```python
from build123d import *

# Parameters (mm, degrees)
ESBO_O1_R                = 4.1
ESBO_O1_R_2              = 1.2
RESSALTO_EXTRUS_O1_DEPTH = 1
ESBO_O2_W                = 5
ESBO_O2_H                = 1
RESSALTO_EXTRUS_O2_DEPTH = 22.2
ESBO_O3_R                = 1.2
RESSALTO_EXTRUS_O3_DEPTH = 1
FILETE1_R                = 1
BODY_MOVE_COPY2_ANGLE    = 90


with BuildPart() as part:
    # Esboço1 → Ressalto-extrusão1 (new body)
    with BuildSketch(Plane(origin=(0, 0, 0), x_dir=(1, 0, 0), z_dir=(0, 1, 0))):
        with BuildLine():
            Line((-2.5, 15), (-2.5, 12.247448714))
            ThreePointArc((-2.5, 12.247448714), (-10.825317547, 6.25), (-11.856601718, -3.958660847))
            Line((-11.856601718, -3.958660847), (-14.240381057, -5.334936491))
            Line((-14.240381057, -5.334936491), (-11.740381057, -9.665063509))
            Line((-11.740381057, -9.665063509), (-9.356601718, -8.288787866))
            ThreePointArc((-9.356601718, -8.288787866), (0, -12.5), (9.356601718, -8.288787866))
            Line((9.356601718, -8.288787866), (11.740381057, -9.665063509))
            Line((11.740381057, -9.665063509), (14.240381057, -5.334936491))
            Line((14.240381057, -5.334936491), (11.856601718, -3.958660847))
            ThreePointArc((11.856601718, -3.958660847), (10.825317547, 6.25), (2.5, 12.247448714))
            Line((2.5, 12.247448714), (2.5, 15))
            Line((2.5, 15), (-2.5, 15))
        make_face()
        with Locations(Location((0, 0, 0), (0, 0, 270))):
            Circle(ESBO_O1_R, mode=Mode.SUBTRACT)
        with Locations(Location((0, 6.75, 0), (0, 0, 270))):
            Circle(ESBO_O1_R_2, mode=Mode.SUBTRACT)
        with Locations(Location((5.845671476, -3.375, 0), (0, 0, 270))):
            Circle(ESBO_O1_R_2, mode=Mode.SUBTRACT)
        with Locations(Location((-5.845671476, -3.375, 0), (0, 0, 270))):
            Circle(ESBO_O1_R_2, mode=Mode.SUBTRACT)
    extrude(amount=RESSALTO_EXTRUS_O1_DEPTH)

    # Esboço2 → Ressalto-extrusão2 (add)
    with BuildSketch(Plane.XZ):
        with Locations((0, -14.5)):
            Rectangle(ESBO_O2_W, ESBO_O2_H)
        Polygon((-10.874355653, 9.165063509), (-11.740381057, 9.665063509), (-14.240381057, 5.334936491), (-13.374355653, 4.834936491), align=None)
        Polygon((13.374355653, 4.834936491), (14.240381057, 5.334936491), (11.740381057, 9.665063509), (10.874355653, 9.165063509), align=None)
    extrude(amount=RESSALTO_EXTRUS_O2_DEPTH)

    # Esboço3 → Ressalto-extrusão3 (add)
    # profile 1 of 3: a face of its own
    with BuildSketch(Plane.XZ.offset(22.2)):
        with BuildLine():
            Line((2.5, -15), (2.5, -17.5))
            ThreePointArc((2.5, -17.5), (0, -20), (-2.5, -17.5))
            Line((-2.5, -17.5), (-2.5, -15))
            Line((-2.5, -15), (2.5, -15))
        make_face()
        with Locations(Location((0, -17.5, 0), (0, 0, 270))):
            Circle(ESBO_O3_R, mode=Mode.SUBTRACT)
    # profile 2 of 3: a face of its own
    with BuildSketch(Plane.XZ.offset(22.2)):
        with BuildLine():
            Line((-11.740381057, 9.665063509), (-13.905444566, 10.915063509))
            ThreePointArc((-13.905444566, 10.915063509), (-17.320508076, 10), (-16.405444566, 6.584936491))
            Line((-16.405444566, 6.584936491), (-14.240381057, 5.334936491))
            Line((-14.240381057, 5.334936491), (-11.740381057, 9.665063509))
        make_face()
        with Locations(Location((-15.155444566, 8.75, 0), (0, 0, 270))):
            Circle(ESBO_O3_R, mode=Mode.SUBTRACT)
    # profile 3 of 3: a face of its own
    with BuildSketch(Plane.XZ.offset(22.2)):
        with BuildLine():
            Line((14.240381057, 5.334936491), (16.405444566, 6.584936491))
            ThreePointArc((16.405444566, 6.584936491), (17.320508076, 10), (13.905444566, 10.915063509))
            Line((13.905444566, 10.915063509), (11.740381057, 9.665063509))
            Line((11.740381057, 9.665063509), (14.240381057, 5.334936491))
        make_face()
        with Locations(Location((15.155444566, 8.75, 0), (0, 0, 270))):
            Circle(ESBO_O3_R, mode=Mode.SUBTRACT)
    extrude(amount=-RESSALTO_EXTRUS_O3_DEPTH)

    # Filete1
    filete1_edges = [part.edges().sort_by_distance(p)[0] for p in [
        (11.856601718, 0.5, 3.958660847),
        (2.5, 0.5, -12.247448714),
        (-2.5, 0.5, -12.247448714),
        (-11.856601718, 0.5, 3.958660847),
        (9.356601718, 0.5, 8.288787866),
        (-9.356601718, 0.5, 8.288787866),
    ]]
    fillet(filete1_edges, radius=FILETE1_R)


with BuildPart() as part_1:
    # Body-Move/Copy2: moved
    add(part.part.rotate(Axis((0, -10.6, -3.75), (1, 0, 0)), BODY_MOVE_COPY2_ANGLE))


solid = part_1.part
```
The listing builds one solid part. Answer for the finished solid, in the listing's coordinates (mm). A direction names the side the tool comes from. Coordinates: 2 decimals unless noted, no trailing zeros. Loops run counter-clockwise (first coordinate to the right, second up) from the corner with the lowest first, then second, coordinate; pieces in that order, holes last. Notation, with made-up numbers: (42.25, 45.5) - (88.25, 45.5) arc R10 ccw to (88.25, 49.5) - close; hole circle Ø1 at (-20, -31). An arc over 180 degrees is marked (long way). Use a Markdown table: item, result. Add a question column.
1) Find the intervals of material crossed by line 1 (X direction, y = -14.35, z = 7.25); line 2 (Z direction, x = 9, y = -18); line 3 (X direction, y = -23.1, z = -14.8), in increasing order.
2) Given pin 1 (2 mm diameter, centred on y = 1, z = 0, fed in from -X); pin 2 (2 mm diameter, centred on x = 0, y = 3.15, fed in from -Z); pin 3 (1.5 mm diameter, centred on x = -0.5, y = 3.5, fed in from +Z); pin 4 (1.5 mm diameter, centred on x = 0.5, y = -8.5, fed in from -Z), each flat-ended and moving along its own axis, determine where each tip first touches the part or whether it passes through.
3) The mould has two halves that part along Y. Classify faces 1 (the cylindrical face through (10.893, -8.219, 7.343)), 2 (the flat face through (0, 0.65, -3)), 3 (the cylindrical face through (-5.793, -16.526, 7.343)), 4 (the flat face through (0, -19, 6.85)): released by +Y, released by -Y, zero draft, split by the parting line, or undercut.
4) The part is cut by section B-B, the plane x = 0. Give the vertices of the cut face in (y, z), and give its area (3 significant figures).
5) The part is cut by section C-C, the plane z = 2.5. Give the vertices of the cut face in (x, y).
6) For faces 5 (the flat face through (12.107, -21.38, -4.095)), 6 (the flat face through (-13.01, -21.82, -3.41)), 7 (the cylindrical face through (0.05, 5.65, -14.86)), determine the directions among +Z, -Z, +X, -X, +Y, -Y from which every point of the face is accessible in a straight line to the end or side of a thin tool.
7) The part is cut by section D-D, the plane x = -7.5. Give the vertices of the cut face in (y, z), and give its area (3 significant figures).
8) The part is cut by section A-A, the plane y = -14.35. Give the vertices of the cut face in (x, z).
Here are the results:
| question | item | result |
|---|---|---|
| 1 | line 1 | x = -12.5 to -4.1, 4.1 to 12.5 |
| 1 | line 2 | z = 6.85 to 7.85 |
| 1 | line 3 | x = -17.66 to -16.36, -13.96 to -11.11, 11.11 to 13.96, 16.36 to 17.66 |
| 2 | pin 1 | stops at x = -2.5 |
| 2 | pin 2 | passes through |
| 2 | pin 3 | stops at z = -14.35 |
| 2 | pin 4 | stops at z = 6.85 |
| 3 | face 1 | undercut |
| 3 | face 2 | released by +Y |
| 3 | face 3 | undercut |
| 3 | face 4 | zero draft |
| 4 | outline | (-26.85, 6.85) - (-18.45, 6.85) - (-18.45, 7.85) - (-26.85, 7.85) - close; (-10.25, 6.85) - (-8.8, 6.85) - (-8.8, 7.85) - (-10.25, 7.85) - close; (-6.4, 6.85) - (-0.35, 6.85) - (-0.35, -15.35) - (1.95, -15.35) - (1.95, -14.35) - (0.65, -14.35) - (0.65, 7.85) - (-6.4, 7.85) - close; (4.35, -15.35) - (5.65, -15.35) - (5.65, -14.35) - (4.35, -14.35) - close |
| 4 | area | 41.7 mm^2 |
| 5 | outline | (-14.24, -19.68) - (-11.74, -24.02) - (-10.87, -23.52) - (-13.37, -19.18) - close; (-2.5, -0.35) - (2.5, -0.35) - (2.5, 0.65) - (-2.5, 0.65) - close; (10.87, -23.52) - (11.74, -24.02) - (14.24, -19.68) - (13.37, -19.18) - close |
| 6 | face 5 | -Z, +Y |
| 6 | face 6 | +Z, -X, -Y |
| 6 | face 7 | +Z, -Z, +Y |
| 7 | outline | (-24.35, 6.85) - (-4.35, 6.85) - (-4.35, 7.85) - (-24.35, 7.85) - close |
| 7 | area | 20.0 mm^2 |
| 8 | outline | (-12.5, 6.85) - (-4.1, 6.85) - (-4.1, 7.85) - (-12.5, 7.85) - close; (4.1, 6.85) - (12.5, 6.85) - (12.5, 7.85) - (4.1, 7.85) - close |
